from build123d import *

# Parameters (mm, degrees)
SKETCH1_R                = 2.75
BOSS_EXTRUDE1_DEPTH      = 8
BOSS_EXTRUDE2_DEPTH      = 5
BOSS_EXTRUDE2_DEPTH_BACK = 5
CUT_EXTRUDE1_DEPTH       = 2.5
CUT_EXTRUDE2_DEPTH       = 2.5
CUT_EXTRUDE3_DEPTH       = 3.5


with BuildPart() as part:
    # Sketch1 → Boss-Extrude1 (new body)
    with BuildSketch(Plane(origin=(0, 0, 0), x_dir=(1, 0, 0), z_dir=(0, 1, 0))):
        with BuildLine():
            Line((-19.5, -15.5), (19.5, -15.5))
            ThreePointArc((19.5, -15.5), (23.742640687, -13.742640687), (25.5, -9.5))
            Line((25.5, -9.5), (25.5, 9.5))
            ThreePointArc((25.5, 9.5), (23.742640687, 13.742640687), (19.5, 15.5))
            Line((19.5, 15.5), (-19.5, 15.5))
            ThreePointArc((-19.5, 15.5), (-23.742640687, 13.742640687), (-25.5, 9.5))
            Line((-25.5, 9.5), (-25.5, -9.5))
            ThreePointArc((-25.5, -9.5), (-23.742640687, -13.742640687), (-19.5, -15.5))
        make_face()
        with Locations((19, 9)):
            Circle(SKETCH1_R, mode=Mode.SUBTRACT)
        with Locations((19, -9)):
            Circle(SKETCH1_R, mode=Mode.SUBTRACT)
        with Locations((-19, 9)):
            Circle(SKETCH1_R, mode=Mode.SUBTRACT)
        with Locations((-19, -9)):
            Circle(SKETCH1_R, mode=Mode.SUBTRACT)
    extrude(amount=BOSS_EXTRUDE1_DEPTH)

    # Sketch2 → Boss-Extrude2 (add, two sides)
    with BuildSketch(Plane(origin=(0, 0, 0), x_dir=(0, 0, -1), z_dir=(1, 0, 0))) as boss_extrude2_sk:
        with BuildLine():
            Line((-20.35784849, 27.483766103), (-15.5, 8))
            Line((-15.5, 8), (13.085782237, 8))
            Line((13.085782237, 8), (-2.5, 32))
            ThreePointArc((-2.5, 32), (-9.670789904, 22.789963066), (-20.35784849, 27.483766103))
        make_face()
    extrude(amount=BOSS_EXTRUDE2_DEPTH)
    extrude(boss_extrude2_sk.sketch, amount=-BOSS_EXTRUDE2_DEPTH_BACK)

    # Sketch3 → Cut-Extrude1 (cut)
    with BuildSketch(Plane(origin=(5, 0, 0), x_dir=(0, 0, -1), z_dir=(1, 0, 0))):
        with BuildLine():
            Line((-12.894702583, 19.52726585), (-10.203178684, 9.48236191))
            ThreePointArc((-10.203178684, 9.48236191), (-9.48884989, 8.413293319), (-8.271327032, 8))
            Line((-8.271327032, 8), (3.344242354, 8))
            ThreePointArc((3.344242354, 8), (5.101876579, 9.045682479), (5.02158349, 11.08927807))
            Line((5.02158349, 11.08927807), (-3.061203443, 23.535678478))
            ThreePointArc((-3.061203443, 23.535678478), (-4.395332352, 24.416731692), (-5.948787149, 24.038667007))
            ThreePointArc((-5.948787149, 24.038667007), (-8.400375652, 22.670332023), (-11.135709109, 22.03741995))
            ThreePointArc((-11.135709109, 22.03741995), (-12.60073654, 21.192654231), (-12.894702583, 19.52726585))
        make_face()
    extrude(amount=-CUT_EXTRUDE1_DEPTH, mode=Mode.SUBTRACT)

    # Sketch4 → Cut-Extrude2 (cut)
    with BuildSketch(Plane(origin=(-5, 0, 0), x_dir=(0, 0, -1), z_dir=(1, 0, 0))):
        with BuildLine():
            Line((-12.894702583, 19.52726585), (-10.203178684, 9.48236191))
            ThreePointArc((-10.203178684, 9.48236191), (-9.48884989, 8.413293319), (-8.271327032, 8))
            Line((-8.271327032, 8), (3.344242354, 8))
            ThreePointArc((3.344242354, 8), (5.101876579, 9.045682479), (5.02158349, 11.08927807))
            Line((5.02158349, 11.08927807), (-3.061203443, 23.535678478))
            ThreePointArc((-3.061203443, 23.535678478), (-4.395332352, 24.416731692), (-5.948787149, 24.038667007))
            ThreePointArc((-5.948787149, 24.038667007), (-8.400375652, 22.670332023), (-11.135709109, 22.03741995))
            ThreePointArc((-11.135709109, 22.03741995), (-12.60073654, 21.192654231), (-12.894702583, 19.52726585))
        make_face()
    extrude(amount=CUT_EXTRUDE2_DEPTH, mode=Mode.SUBTRACT)

    # Sketch5 → Revolve1 (revolve)
    with BuildSketch(Plane.XY.offset(12)):
        with BuildLine():
            Line((-7.9, 41), (-7.9, 37))
            Line((-7.9, 37), (7.9, 37))
            Line((7.9, 37), (7.9, 41))
            ThreePointArc((7.9, 41), (7.607106781, 41.707106781), (6.9, 42))
            Line((6.9, 42), (-6.9, 42))
            ThreePointArc((-6.9, 42), (-7.607106781, 41.707106781), (-7.9, 41))
        make_face()
    revolve(axis=Axis((7.9, 32, 12), (-1, 0, 0)))

    # Sketch6 → Cut-Extrude3 (cut)
    with BuildSketch(Plane(origin=(0, 0, 0), x_dir=(1, 0, 0), z_dir=(0, 1, 0))):
        with BuildLine():
            Line((-20.5, 0.013899622), (-20.5, -0.013899622))
            ThreePointArc((-20.5, -0.013899622), (-19.952966315, -1.388268164), (-18.611111111, -2.010810817))
            ThreePointArc((-18.611111111, -2.010810817), (-14.190149162, -3.914202627), (-12.04334407, -8.222222222))
            ThreePointArc((-12.04334407, -8.222222222), (-11.389061423, -9.490711985), (-10.05572809, -10))
            Line((-10.05572809, -10), (10.05572809, -10))
            ThreePointArc((10.05572809, -10), (11.389061423, -9.490711985), (12.04334407, -8.222222222))
            ThreePointArc((12.04334407, -8.222222222), (14.190149162, -3.914202627), (18.611111111, -2.010810817))
            ThreePointArc((18.611111111, -2.010810817), (19.952966315, -1.388268164), (20.5, -0.013899622))
            Line((20.5, -0.013899622), (20.5, 0.013899622))
            ThreePointArc((20.5, 0.013899622), (19.952966315, 1.388268164), (18.611111111, 2.010810817))
            ThreePointArc((18.611111111, 2.010810817), (14.190149162, 3.914202627), (12.04334407, 8.222222222))
            ThreePointArc((12.04334407, 8.222222222), (11.389061423, 9.490711985), (10.05572809, 10))
            Line((10.05572809, 10), (-10.05572809, 10))
            ThreePointArc((-10.05572809, 10), (-11.389061423, 9.490711985), (-12.04334407, 8.222222222))
            ThreePointArc((-12.04334407, 8.222222222), (-14.190149162, 3.914202627), (-18.611111111, 2.010810817))
            ThreePointArc((-18.611111111, 2.010810817), (-19.952966315, 1.388268164), (-20.5, 0.013899622))
        make_face()
    extrude(amount=CUT_EXTRUDE3_DEPTH, mode=Mode.SUBTRACT)


solid = part.part
Here's how the part is built. I have some questions about the finished solid (model axes, mm). A direction names the side the tool comes from. Coordinates: 2 decimals unless noted, no trailing zeros. Loops run counter-clockwise (first coordinate to the right, second up) from the corner with the lowest first, then second, coordinate; pieces in that order, holes last. Notation, with made-up numbers: (80, -2) -> (88, -2) arc R24 ccw to (88, 36) -> close; hole circle Ø3 at (59.5, -26). An arc over 180 degrees is marked (long way). Use one line per item in the form item = value. Start each with the question number.
(1) If we section it at C-C (z = -11): Please give me the cut outline in (x, y), then the cut area to 3 significant figures.
(2) On a 3-axis mill with a long thin cutter (end or side, diameter ignored), from which of +Z, -Z, +X, -X, +Y, -Y can I reach the whole of each face in a straight line? I mean faces 5 (the face through (7.9, 28, 16)), 6 (the face through (3.768, 24.413, 4.373)), 7 (the face through (-14.24, 1.73, 3.87)), 8 (the face through (-3.77, 14.58, 11.57)). Say none if no direction works.
(3) If we section it at D-D (y = 14.5): Please give me the cut outline in (x, z), then the cut area to 3 significant figures.
(4) Will these pins go through, and if not, where does the flat tip stop? pin 1 (3 mm diameter, centred on x = 3, y = 1, fed in from +Z); pin 2 (13 mm diameter, centred on y = 19.5, z = 14, fed in from -X); pin 3 (7 mm diameter, centred on x = 19, z = -9, fed in from +Y); pin 4 (5.5 mm diameter, centred on y = 24.5, z = -7, fed in from +X).
(5) We'd pull the mould along X, two halves only. Please class faces 1 (the face through (11.4, 1.73, -9.48)), 2 (the face through (14.24, 1.73, -3.87)), 3 (the face through (3.77, 21.21, 12.59)), 4 (the face through (-5, 15, 14)): pulls with the +X half, pulls with the -X half, needs draft (parallel to the pull), parting line crosses it, or undercut.
(6) If we section it at B-B (x = -1.5): Please give me the cut outline in (y, z).
(7) Please list where these lines run through material, in increasing order: line 1 along X through (y, z) = (4, -9); line 2 along Y through (x, z) = (-0.5, 12); line 3 along X through (y, z) = (3, 9).
(8) If we section it at A-A (y = 32): Please give me the cut outline in (x, z), then the cut area to 3 significant figures.
Verdict:
q1.outline = (-25.31, 0) -> (-20.89, 0) -> (-20.89, 8) -> (-25.31, 8) -> close; (-17.11, 0) -> (17.11, 0) -> (17.11, 8) -> (5, 8) -> (5, 11.21) -> (-5, 11.21) -> (-5, 8) -> (-17.11, 8) -> close; (20.89, 0) -> (25.31, 0) -> (25.31, 8) -> (20.89, 8) -> close
q1.area = 377 mm²
q2.face_5 = +Z, -Z, +X, +Y
q2.face_6 = +X
q2.face_7 = -Y
q2.face_8 = -X
q3.outline = (-5, -8.86) -> (5, -8.86) -> (5, -2.81) -> (2.5, -2.81) -> (2.5, 11.55) -> (5, 11.55) -> (5, 17.12) -> (-5, 17.12) -> (-5, 11.55) -> (-2.5, 11.55) -> (-2.5, -2.81) -> (-5, -2.81) -> close
q3.area = 188 mm²
q4.pin_1 = 15.5
q4.pin_2 = -7.9
q4.pin_3 = 8
q4.pin_4 = through
q5.face_1 = undercut
q5.face_2 = undercut
q5.face_3 = needs draft
q5.face_4 = pulls with the -X half
q6.outline = (0, -15.5) -> (8, -15.5) -> (8, -13.09) -> (31.27, 2.03) arc R10 ccw (long way) to (25.98, 19.98) -> (8, 15.5) -> (0, 15.5) -> (0, 10) -> (3.5, 10) -> (3.5, -10) -> (0, -10) -> close; hole circle Ø10 at (32, 12)
q7.line_1 = -25.5 to -21.75, -16.25 to 16.25, 21.75 to 25.5
q7.line_2 = 0 to 27, 37 to 42
q7.line_3 = -25.5 to -21.75, -16.25 to -11.79, 11.79 to 16.25, 21.75 to 25.5
q8.outline = (-7.9, 3) arc R1 ccw to (-6.9, 2) -> (6.9, 2) arc R1 ccw to (7.9, 3) -> (7.9, 7) -> (-7.9, 7) -> close; (-7.9, 17) -> (7.9, 17) -> (7.9, 21) arc R1 ccw to (6.9, 22) -> (-6.9, 22) arc R1 ccw to (-7.9, 21) -> close
q8.area = 157 mm²
